Design review of the part shown in the three views and the two pictorial views. Dimensions are in mm from the part's minimum x, y and z. A direction names the side the tool comes from. Coordinates: 2 decimals unless noted, no trailing zeros. Order: outer loops, then holes, each group sorted by start corner. A loop starts at its lowest first (then second) coordinate and runs counter-clockwise, first axis right, second up. Notation, with made-up numbers: (2, 74.5) -> (28, 74.5) arc R28 cw to (28, 101.5) -> close; hole circle Ø2 at (40, -27.75). An arc over 180 degrees is marked (long way). Write item = value, one per line. Start each with the question number.
1) Insertion check: pin 1 Ø6.5 at (x, z) = (8.5, 22) entering from -Y; pin 2 Ø13.5 at (x, z) = (44, 22.5) entering from +Y; pin 3 Ø1.5 at (x, z) = (7, 44) entering from -Y; pin 4 Ø1.5 at (x, z) = (43.5, 45) entering from +Y. Each pin has a flat end and moves straight along its axis. Give the tip position at first contact, or say it passes through.
2) Consider section D-D on y = 17. Give the boundary of the cut face in (x, z), and give its area (3 significant figures).
3) Consider section B-B on x = 30. Give the boundary of the cut face in (y, z), and give its area (3 significant figures).
4) Draft analysis for pull direction Y (two halves, no side actions). For the marked faces 6, 7 and 8, state which applies: +Y half, -Y half, draft (parallel to the pull), parting line (faces both ways), or undercut.
5) Consider section A-A on z = 12. Give the boundary of the cut face in (x, y).
6) Consider section C-C on z = 28.5. Give the boundary of the cut face in (x, y), and give its area (3 significant figures).
7) Machinability: for the marked faces 1, 2, 3, 4 and 5, which of the approach directions +Z, -Z, +X, -X, +Y, -Y give a long, thin tool a straight path to every point of the face, cutting with its end or side? Answer none if there is none.
8) Wall thickness on probe 1 along Y at (x, z) = (48.5, 38); probe 2 along X at (y, z) = (17, 9.25); probe 3 along X at (y, z) = (17.5, 5.5): over which ranges is each line inside the solid? List them lowest first. Write a range as [from, to].
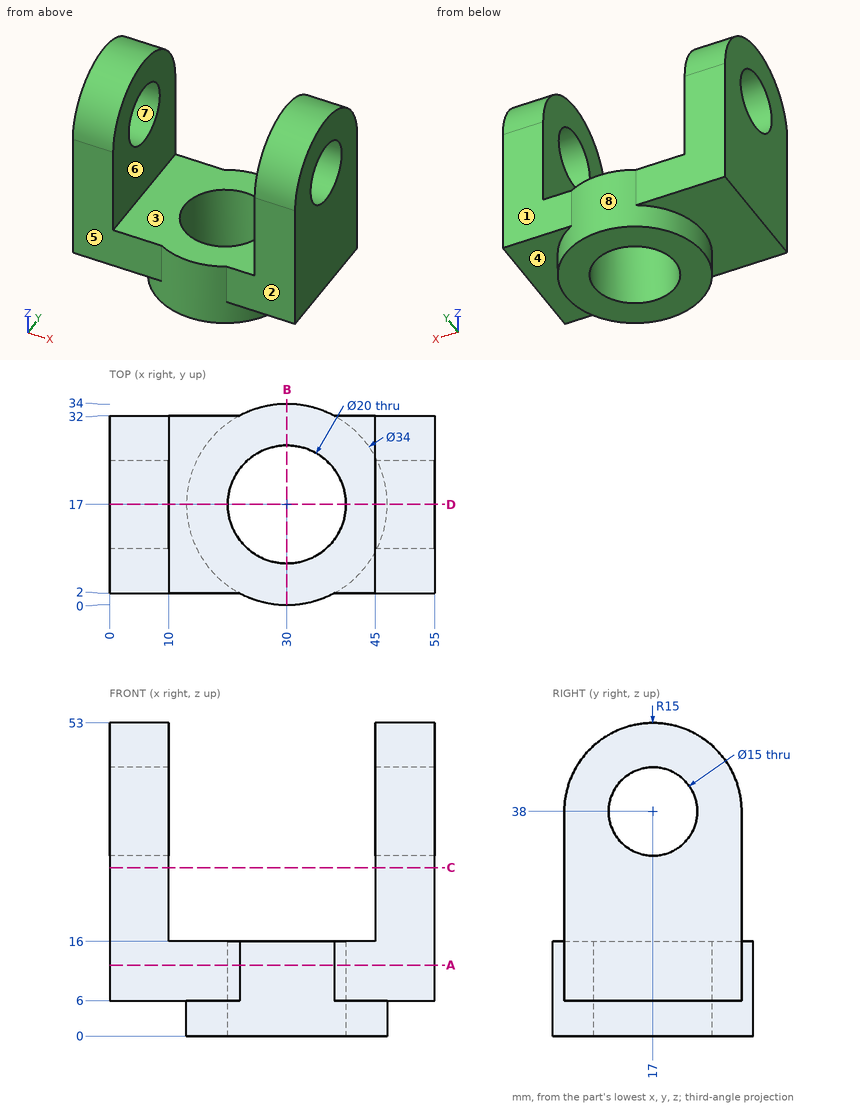
Answer sheet:
q1.pin_1 = 2
q1.pin_2 = 32
q1.pin_3 = 2.95
q1.pin_4 = through
q2.outline = (0, 6) -> (13, 6) -> (13, 0) -> (20, 0) -> (20, 16) -> (10, 16) -> (10, 30.5) -> (0, 30.5) -> close; (0, 45.5) -> (10, 45.5) -> (10, 53) -> (0, 53) -> close; (40, 0) -> (47, 0) -> (47, 6) -> (55, 6) -> (55, 30.5) -> (45, 30.5) -> (45, 16) -> (40, 16) -> close; (45, 45.5) -> (55, 45.5) -> (55, 53) -> (45, 53) -> close
q2.area = 874 mm2
q3.outline = (0, 0) -> (7, 0) -> (7, 16) -> (0, 16) -> close; (27, 0) -> (34, 0) -> (34, 16) -> (27, 16) -> close
q3.area = 224 mm2
q4.face_6 = draft
q4.face_7 = undercut
q4.face_8 = parting line
q5.outline = (0, 2) -> (22, 2) arc R17 ccw to (38, 2) -> (55, 2) -> (55, 32) -> (38, 32) arc R17 ccw to (22, 32) -> (0, 32) -> close; hole circle Ø20 at (30, 17)
q6.outline = (0, 2) -> (10, 2) -> (10, 32) -> (0, 32) -> close; (45, 2) -> (55, 2) -> (55, 32) -> (45, 32) -> close
q6.area = 600 mm2
q7.face_1 = +Z, -Z, +X, +Y
q7.face_2 = +Z, -Z, +X, -Y
q7.face_3 = +Z, +Y, -Y
q7.face_4 = -Z, +X
q7.face_5 = +Z, -Z, -X, -Y
q8.probe_1 = [2, 9.5], [24.5, 32]
q8.probe_2 = [0, 20], [40, 55]
q8.probe_3 = [13.01, 20.01], [39.99, 46.99]
